Autodesk Inventor part; units mm, degrees
ref_plane "YZ Plane" through (0, 0, 0) normal (1, 0, 0) x (0, 1, 0)
ref_plane "XZ Plane" through (0, 0, 0) normal (0, 1, 0) x (-1, 0, 0)
ref_plane "XY Plane" through (0, 0, 0) normal (0, 0, 1) x (1, 0, 0)
sketch "Sketch1" plane through (0, 0, 0) normal (1, 0, 0) x (0, 1, 0)
  circle A0 centre (0, 0) radius 11
  line L0 (-12.7, 12.7) -> (12.7, 12.7)
  line L1 (12.7, 12.7) -> (12.7, -12.7)
  line L2 (12.7, -12.7) -> (-12.7, -12.7)
  line L3 (-12.7, -12.7) -> (-12.7, 12.7)
  line L4 (-12.7, 12.7) -> (12.7, -12.7) construction
  line L5 (12.7, 12.7) -> (-12.7, -12.7) construction
  line L6 (-9.525, 9.525) -> (9.525, 9.525) construction
  line L7 (9.525, 9.525) -> (9.525, -9.525) construction
  line L8 (9.525, -9.525) -> (-9.525, -9.525) construction
  line L9 (-9.525, -9.525) -> (-9.525, 9.525) construction
  line L10 (-9.525, 9.525) -> (9.525, -9.525) construction
  line L11 (9.525, 9.525) -> (-9.525, -9.525) construction
  circle A1 centre (9.525, 9.525) radius 1.7526
  circle A2 centre (-9.525, 9.525) radius 1.7526
  circle A3 centre (-9.525, -9.525) radius 1.7526
  circle A4 centre (9.525, -9.525) radius 1.7526
  dimension "d0" = 22
  dimension "d1" = 25.4
  dimension "d2" = 25.4
  dimension "d3" = 19.05
  dimension "d4" = 19.05
  dimension "d5" = 3.5052
  dimension "d8" = 360
extrude "Extrusion1" add sketch "Sketch1" along normal blind 16.8
sketch "Sketch2" plane through (0, 12.7, 12.7) normal (0, 1, 0) x (1, 0, 0)
  circle A0 centre (12.0375, -3.175) radius 4.7625
  circle A1 centre (12.0375, -3.175) radius 3.175
  line L0 (0, 0) -> (16.8, 0)
  line L1 (16.8, 25.4) -> (16.8, 0)
  line L2 (0, 12.7) -> (16.8, 12.7) construction
  line L3 (16.8, -12.7833) -> (16.8, 0)
  circle A2 centre (12.0375, 28.575) radius 4.7625
  circle A3 centre (12.0375, 28.575) radius 3.175
  line L4 (0, 25.4) -> (16.8, 25.4)
  line L5 (16.8, 38.1833) -> (16.8, 25.4)
  line L6 (0, 25.4) -> (16.8, 25.4)
  line L7 (0, 25.4) -> (16.8, 38.1833)
  line L8 (0, 0) -> (16.8, -12.7833)
  point P0 (16.8, -3.175)
  point P1 (16.8, 28.575)
  point P2 (15.5873, 25.4)
  point P3 (8.4877, 25.4)
  point P4 (9.1536, -6.9651)
  point P5 (8.4877, 0)
  point P6 (15.5873, 0)
  dimension "d12" = 9.525
  dimension "d13" = 6.35
extrude "Extrusion2" add sketch "Sketch2" against normal up to surface (25.4 mm away) contours A0 L0 | L3 L8 A0 | A0 L0 L3 | L8 L0 A0 | A2 L4 | L5 L4 A2 | A2 L7 L5 | A2 L4 L7 | A2 L4 picked at (16.2227, -3.5628)
thicken "Thicken1" operation cut thickness 0.254 both sides no extend neighbours no toward (0.9967573, 0, 0.0804666) faces at (15.2022, -4.2333, 16.1305)
thicken "Thicken2" operation cut thickness 0.254 both sides no extend neighbours no toward (0.9870503, 0, -0.1604113) faces at (15.1714, 4.2333, -16.3843)
fillet "Fillet4" radius 3.175 2 edges at (16.8, 0, 25.4833) (16.8, 0, -25.4833)
properties part number "Motor Sleeve" material "UHMW, Black"
CAD build for the part. Positions are in the model's coordinates, mm. A direction names the side the tool comes from. Give positions to 0.01 mm unless a question says otherwise; leave off trailing zeros. Order: outer loops, then holes, each group sorted by start corner. A loop starts at its lowest first (then second) coordinate and runs counter-clockwise, first axis right, second up.
(1) Tool access for faces 4 (the flat face through (8, -12.7, 0)), 5 (the cylindrical face through (12.02, 9.535, -11.113)): list every direction of +Z, -Z, +X, -X, +Y, -Y with a clear straight run to the whole face (end or side of a thin tool).
(2) Flat gauge pins, fed straight in: pin 1 (4 mm diameter, centred on x = 11, y = -9, fed in from -Z); pin 2 (1 mm diameter, centred on x = 5, y = 4.5, fed in from -Z) (3 decimals); pin 3 (4 mm diameter, centred on x = 5, y = 8.5, fed in from +Z). Where does each tip first touch, or does it go through?
(3) Mould opens along Y. For faces 1 (the cylindrical face through (8.282, 9.145, -7.814)), 2 (the flat face through (0, -0.2, 11.5)), 3 (the flat face through (8, 12.7, 0)) say: released by +Y, released by -Y, zero draft, split by the parting line, or undercut.
(4) Saw through at C-C, the plane x = 10.25. Give the cut face in (y, z) (3 decimals).
(5) Drill centre lines: L1, parallel to Z at x = 12, y = 5; L2, parallel to Y at x = 13.25, z = -9.5; L3, parallel to Z at x = 14.25, y = 4.25. Where is each one in solid material? Low to high.
(6) Saw through at B-B, the plane y = 6. State how many separate pieces and enclosed holes the cut face has, then the cut area to 3 significant figures.
(7) Saw through at A-A, the plane z = 0. Give the cut face in (x, y).
Results found:
1. face 4: +Z, -Z, +X, -X, -Y
1. face 5: none
2. pin 1: stops at z = -22.19
2. pin 2: stops at z = -16.885
2. pin 3: stops at z = 18.03
3. face 1: undercut
3. face 2: zero draft
3. face 3: released by +Y
4. outline: (-12.7, -20.499) - (12.7, -20.499) - (12.7, -18.801) - (-12.7, -18.801) - close; (-12.7, -12.949) - (12.7, -12.949) - (12.7, 12.949) - (-12.7, 12.949) - close; (-12.7, 18.801) - (12.7, 18.801) - (12.7, 20.499) - (-12.7, 20.499) - close; hole circle Ø3.505 at (-9.525, -9.525); hole circle Ø3.505 at (-9.525, 9.525); hole circle Ø22 at (0, 0); hole circle Ø3.505 at (9.525, -9.525); hole circle Ø3.505 at (9.525, 9.525)
5. L1: z = -21.81 to -19.3, -12.45 to -9.8, 9.8 to 12.45, 19.3 to 21.81
5. L2: y = -12.7 to -11.28, -7.77 to -5.55, 5.55 to 7.77, 11.28 to 12.7
5. L3: z = -22.19 to -18.49, -13.26 to -10.15, 10.15 to 13.26, 18.49 to 22.19
6. separate pieces: 2
6. enclosed holes: 2
6. area: 240 mm2
7. outline: (0, -12.7) - (16.8, -12.7) - (16.8, -11) - (0, -11) - close; (0, 11) - (16.8, 11) - (16.8, 12.7) - (0, 12.7) - close
